Geometry: see drawing. Coordinates: mm, zero at the bounding-box minimum. A direction names the side the tool comes from. Give positions to 0.01 mm unless a question says otherwise; leave off trailing zeros. Write each loop counter-clockwise with the first axis right and the second up, starting at its lowest first coordinate (ties: lowest second). Pieces come first, ordered by that corner, then holes. Notation, with made-up numbers: M 75,-7.75 L 91,-7.75 A25 ccw 91,27.25 Z; hole C -14.75,33 d1. An arc over 180 degrees is marked long. Answer as a JSON object with one key per item and string values. Group by question number.
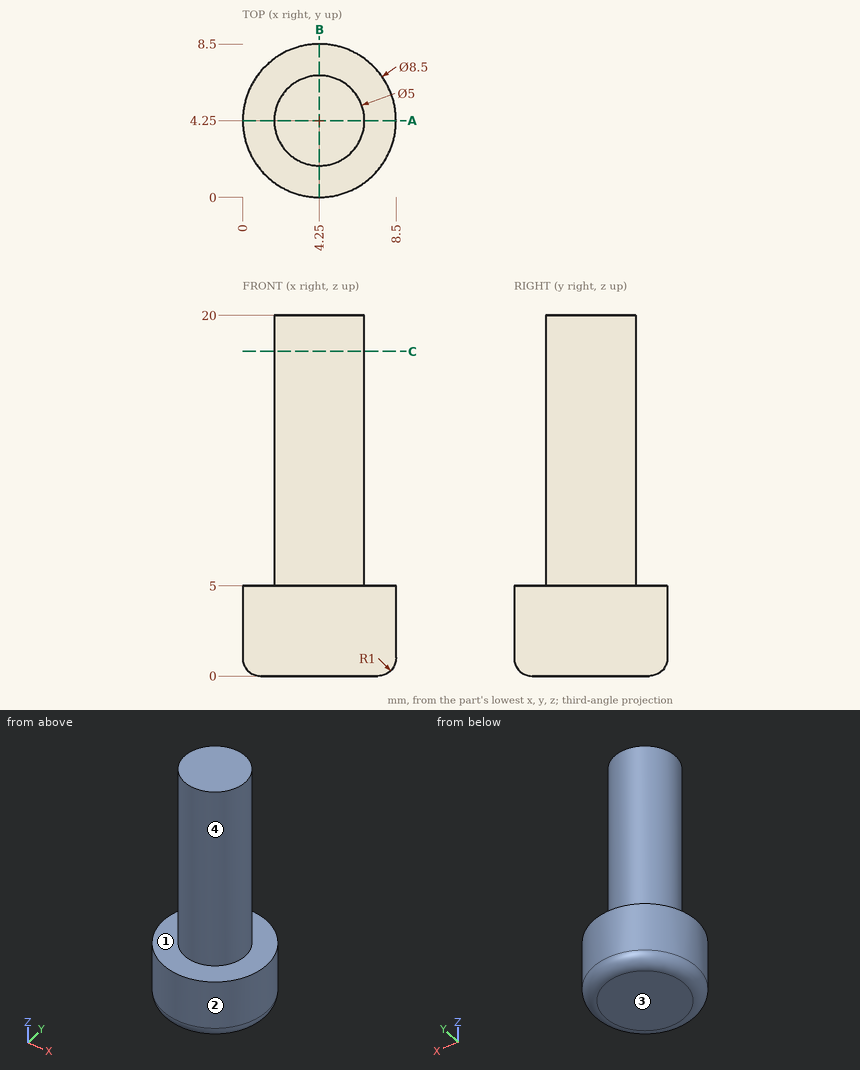
(1) Pull-direction query (Y, two-part tool) for the marked faces 1 and 2; classes: pulls with the +Y half, pulls with the -Y half, needs draft (parallel to the pull), parting line crosses it, or undercut.
(2) Contact query for flat-ended pins moving along their axis: pin 1 Ø3 at (x, z) = (6.5, 8) entering from +Y; pin 2 Ø3 at (y, z) = (4.5, 9) entering from +X. Output: stop coordinate, or through.
(3) Access query for the marked faces 3 and 4. Directions: +Z, -Z, +X, -X, +Y, -Y. A direction counts if a zero-diameter tool reaches every point of the face in a straight line with its end or side. Return the directions, or none.
(4) Ray query, L1, parallel to Z at x = 4.75, y = 1.25; L2, parallel to Z at x = 5, y = 0.75; L3, parallel to X at y = 3.75, z = 16. Return the intervals inside material, ascending. Write a range as [from, to].
(5) Section A-A, the plane y = 4.25. Return loops of the section in (x, z), plus the area to 3 significant figures.
(6) Section C-C, the plane z = 18. Return loops of the section in (x, y), plus the area to 3 significant figures.
Reported:
{
 "1": {"face 1": "needs draft", "face 2": "parting line crosses it"},
 "2": {"pin 1": "stops at y = 6.63", "pin 2": "stops at x = 6.75"},
 "3": {"face 3": "-Z, +X, -X, +Y, -Y", "face 4": "+Z"},
 "4": {"L1": "z = [0, 5]", "L2": "z = [0.06, 5]", "L3": "x = [1.8, 6.7]"},
 "5": {"outline": "M 0,1 A1 ccw 1,0 L 7.5,0 A1 ccw 8.5,1 L 8.5,5 L 6.75,5 L 6.75,20 L 1.75,20 L 1.75,5 L 0,5 Z", "area": "117 mm2"},
 "6": {"outline": "C 4.25,4.25 d5", "area": "19.6 mm2"}
}
